```python
from build123d import *

# Parameters (mm, degrees)
EXTRUDE_THIN1_DEPTH        = 193.5
CONVERT_SOLID1_START       = -193.5
CONVERT_SOLID1_DEPTH       = 387
CONVERT_SOLID1_2_DEPTH     = 387
FILLET1_R                  = 2
F_6_5_6_5_DIAMETER_HOLE1_D = 6.5


# Read off the part's stored shape, not the designer's step: Convert-Solid1
with BuildPart() as part:
    # Sketch1 → Extrude-Thin1 (new, symmetric)
    with BuildSketch(Plane.XY):
        Polygon((-155, -22), (-155, 0), (155, 0), (155, -22), (151, -22), (151, -4), (-151, -4), (-151, -22), align=None)
    extrude(amount=EXTRUDE_THIN1_DEPTH, both=True)

    # Convert-Solid1 outline → Convert-Solid1 (cut)
    with BuildSketch(Plane.XY.offset(CONVERT_SOLID1_START)):
        with BuildLine():
            Line((155, 0), (149, 0))
            ThreePointArc((149, 0), (153.242640687, -1.757359313), (155, -6))
            Line((155, -6), (155, 0))
        make_face()
        with BuildLine():
            ThreePointArc((-155, -6), (-153.242640687, -1.757359313), (-149, 0))
            Line((-149, 0), (-155, 0))
            Line((-155, 0), (-155, -6))
        make_face()
    extrude(amount=CONVERT_SOLID1_DEPTH, mode=Mode.SUBTRACT)

    # Convert-Solid1 2 outline → Convert-Solid1 2 (add)
    with BuildSketch(Plane.XY.offset(CONVERT_SOLID1_START)):
        with BuildLine():
            Line((151, -4), (149, -4))
            ThreePointArc((149, -4), (150.414213562, -4.585786438), (151, -6))
            Line((151, -6), (151, -4))
        make_face()
        with BuildLine():
            ThreePointArc((-151, -6), (-150.414213562, -4.585786438), (-149, -4))
            Line((-149, -4), (-151, -4))
            Line((-151, -4), (-151, -6))
        make_face()
    extrude(amount=CONVERT_SOLID1_2_DEPTH)

    # Fillet1
    fillet1_edges = [part.edges().sort_by_distance(p)[0] for p in [
        (153, -22, 193.5),
        (153, -22, -193.5),
        (-153, -22, -193.5),
        (-153, -22, 193.5),
    ]]
    fillet(fillet1_edges, radius=FILLET1_R)

    # Ø6.5 (6.5) Diameter Hole1 (through all)
    with Locations(Plane(origin=(159, 0, 0), x_dir=(0, 0, -1), z_dir=(1, 0, 0))):
        with Locations((-178.5, -12), (-142.5, -12), (142.5, -12), (178.5, -12)):
            Hole(F_6_5_6_5_DIAMETER_HOLE1_D / 2)


solid = part.part
```
Geometry: final body of the model. Coordinates: model frame, mm. A direction names the side the tool comes from. Round coordinates to 2 decimals unless told otherwise and drop trailing zeros. Order: outer loops, then holes, each group sorted by start corner. A loop starts at its lowest first (then second) coordinate and runs counter-clockwise, first axis right, second up. Notation, with made-up numbers: M 19.25,-22.5 L 30.25,-22.5 A24 ccw 30.25,-2.5 Z; hole C -24.75,88 d8. An arc over 180 degrees is marked long. One line per item, written item: value.
(1) Pin query (flat end, axial travel): P1, Ø4, axis at y = -12, z = 142.5, coming from the -X side; P2, Ø1, axis at x = 0, z = -121.5, coming from the -Y side; P3, Ø1, axis at y = -4, z = 19.5, coming from the -X side. Return the tip coordinate at first contact, or that it passes through.
Result sheet:
P1: through
P2: y = -4
P3: x = -154.81
(2) Reachability of faces 1 (the flat face through (2, -4, 3)), 2 (the flat face through (-1, -2, 193.5)) from +Z, -Z, +X, -X, +Y, -Y: full face, straight path, thin tool, end or side. Return the list, or none.
Result sheet:
face 1: +Z, -Z, -Y
face 2: +Z, +X, -X, +Y, -Y
(3) Pull-direction query (X, two-part tool) for faces 3 (the flat face through (155, -14, 3)), 4 (the flat face through (-151, -14, 3)), 5 (the flat face through (-2, 0, 3)); classes: pulls with the +X half, pulls with the -X half, needs draft (parallel to the pull), parting line crosses it, or undercut.
Result sheet:
face 3: pulls with the +X half
face 4: undercut
face 5: needs draft
(4) Line query: probe 1 along X at (y, z) = (-6.75, 148.5); probe 2 along Y at (x, z) = (-38.5, -107.5); probe 3 along Y at (x, z) = (-153.4, -178.5). Output: solid intervals per line, ascending. Write a range as [from, to].
Result sheet:
probe 1: [-155, -151], [151, 155]
probe 2: [-4, 0]
probe 3: [-22, -15.25], [-8.75, -1.92]
(5) Cut plane A-A (z = -70). Return the cut outline in (x, y).
Result sheet:
outline: M -155,-22 L -151,-22 L -151,-6 A2 cw -149,-4 L 149,-4 A2 cw 151,-6 L 151,-22 L 155,-22 L 155,-6 A6 ccw 149,0 L -149,0 A6 ccw -155,-6 Z
(6) Cut plane B-B (x = 52.5). Return the cut outline in (y, z), and give its area (3 significant figures).
Result sheet:
outline: M -4,-193.5 L 0,-193.5 L 0,193.5 L -4,193.5 Z
area: 1,550 mm2
